Read the model definition and answer for the solid it produces. Units are mm, in the model's axes. A direction names the side the tool comes from. Coordinates: 2 decimals unless noted, no trailing zeros. Loops run counter-clockwise (first coordinate to the right, second up) from the corner with the lowest first, then second, coordinate; pieces in that order, holes last. Notation, with made-up numbers: M 49.5,39.5 L 104.5,39.5 A10 cw 104.5,57.5 Z; hole C 78.25,50 d4. An arc over 180 degrees is marked long. Put each result on its own line as item: value.
from build123d import *

# Parameters (mm, degrees)
F0_R          = 31.75
F0_R_2        = 27.94
F1_DEPTH      = 25.4
F2_R          = 3.175
F3_DEPTH      = 30.48
F3_DEPTH_BACK = 30.48
F4_R          = 31.75
F5_DEPTH      = 5.08


with BuildPart() as f1:
    # F0 (on Top) → F1 (new body)
    with BuildSketch(Plane.XY):
        Circle(F0_R)
        Circle(F0_R_2, mode=Mode.SUBTRACT)
    extrude(amount=F1_DEPTH)

    # F2 (on Right) → F3 (join, two sides)
    with BuildSketch(Plane.YZ) as f3_sk:
        with Locations((0, 20.32)):
            Circle(F2_R)
    extrude(amount=-F3_DEPTH)
    extrude(f3_sk.sketch, amount=F3_DEPTH_BACK)

    # F4 (on Top) → F5 (join)
    with BuildSketch(Plane.XY):
        Circle(F4_R)
    extrude(amount=-F5_DEPTH)


solid = f1.part
1) Find section D-D, the plane y = 9.5. Write down the section's boundary in (x, z), plus the area to 3 significant figures.
Answer list:
outline: M -30.3,-5.08 L 30.3,-5.08 L 30.3,25.4 L 26.28,25.4 L 26.28,0 L -26.28,0 L -26.28,25.4 L -30.3,25.4 Z
area: 512 mm^2
2) Given pin 1 Ø2 at (x, y) = (-8, -9.5) entering from +Z; pin 2 Ø5 at (y, z) = (-16.5, 10.5) entering from -X; pin 3 Ø2 at (y, z) = (-7, 6) entering from +X, each flat-ended and moving along its own axis, determine where each tip first touches the part or whether it passes through.
Answer list:
pin 1: stops at z = 0
pin 2: stops at x = -28.5
pin 3: stops at x = 31.18
3) Which of the six approach directions +Z, -Z, +X, -X, +Y, -Y give full straight-line access (tool end or side, diameter ignored) to faces 4 (the flat face through (0, 0, 0)), 5 (the flat face through (-0.1, -28.1, 25.4))?
Answer list:
face 4: none
face 5: +Z, +X, -X, +Y, -Y
4) Find section C-C, the plane z = 8.5. Write down the section's boundary in (x, y).
Answer list:
outline: C 0,0 d63.5; hole C 0,0 d55.88
5) Determine the mould class of faces 1 (the cylindrical face through (-6.883, -30.995, 10.373)), 2 (the cylindrical face through (-0.39, -0.41, 23.47)), 3 (the flat face through (0, 0, -5.08)) for opening direction Y: released by +Y, released by -Y, zero draft, split by the parting line, or undercut.
Answer list:
face 1: split by the parting line
face 2: undercut
face 3: zero draft
6) Straight lines are drawn through the part: line 1 (X direction, y = -1, z = 11.5); line 2 (X direction, y = -9, z = 19); line 3 (Z direction, x = 15, y = 19). For each, find the intervals that lie inside material, in ascending order. Write a range as [from, to].
Answer list:
line 1: x = [-31.73, -27.92], [27.92, 31.73]
line 2: x = [-30.45, -26.45], [26.45, 30.45]
line 3: z = [-5.08, 0]
7) Find section B-B, the plane x = 0. Write down the section's boundary in (y, z) (3 decimals).
Answer list:
outline: M -31.75,-5.08 L 31.75,-5.08 L 31.75,25.4 L 27.94,25.4 L 27.94,0 L -27.94,0 L -27.94,25.4 L -31.75,25.4 Z; C 0,20.32 d6.35
8) Find section A-A, the plane y = 0. Write down the section's boundary in (x, z) (3 decimals).
Answer list:
outline: M -31.75,-5.08 L 31.75,-5.08 L 31.75,25.4 L 27.94,25.4 L 27.94,23.495 L -27.94,23.495 L -27.94,25.4 L -31.75,25.4 Z; hole M -27.94,0 L 27.94,0 L 27.94,17.145 L -27.94,17.145 Z
